Read the model definition and answer for the solid it produces. Units are mm, in the model's axes. A direction names the side the tool comes from. Give positions to 0.01 mm unless a question says otherwise; leave off trailing zeros. Order: outer loops, then holes, each group sorted by start corner. A loop starts at its lowest first (then second) coordinate and runs counter-clockwise, first axis right, second up. Notation, with made-up numbers: (9.25, 60) -> (34.25, 60) arc R11 cw to (34.25, 64) -> close; hole circle Ø6 at (86.25, 68.5). An arc over 180 degrees is marked (long way). Use one line per item in the form item = value.
```python
from build123d import *

# Parameters (mm, degrees)
SKETCH_1_R                   = 2.6
SM_BASE_FLANGE_1_DEPTH       = 1.2
SM_EDGE_FLANGE_2_DEPTH       = 160
SM_START                     = 1.2
SM_EDGE_FLANGE_2_PROFILE_R   = 5
SM_EDGE_FLANGE_2_PROFILE_R_2 = 2.6
SM_EDGE_FLANGE_2_FLAT_DEPTH  = 1.2


# Sheet-metal steps are written as plain solids
with BuildPart() as part:
    # Sketch 1 → 基体-法兰1 (new body)
    with BuildSketch(Plane.XY):
        with BuildLine():
            Line((-8, 80), (9, 80))
            Line((9, 80), (9, -80))
            Line((9, -80), (-8, -80))
            ThreePointArc((-8, -80), (-9.414213562, -79.414213562), (-10, -78))
            Line((-10, -78), (-10, 78))
            ThreePointArc((-10, 78), (-9.414213562, 79.414213562), (-8, 80))
        make_face()
        with Locations((0, 70)):
            Circle(SKETCH_1_R, mode=Mode.SUBTRACT)
        with Locations((0, -70)):
            Circle(SKETCH_1_R, mode=Mode.SUBTRACT)
    extrude(amount=-SM_BASE_FLANGE_1_DEPTH)

    # 边线-法兰2 bend section (across the edge) → 边线-法兰2 (add)
    with BuildSketch(Plane(origin=(10, -80, 0), x_dir=(-1, 0, 0), z_dir=(0, 1, 0))):
        with BuildLine():
            Line((-1.2, 1), (0, 1))
            ThreePointArc((0, 1), (0.292893219, 0.292893219), (1, 0))
            Line((1, 0), (1, -1.2))
            ThreePointArc((1, -1.2), (-0.555634919, -0.555634919), (-1.2, 1))
        make_face()
    extrude(amount=SM_EDGE_FLANGE_2_DEPTH)

    # 边线-法兰2 profile (on flange) → 边线-法兰2 flat (add)
    with BuildSketch(Plane.YZ.offset(10).offset(SM_START)):
        with BuildLine():
            Line((-80, 15), (-80, 1))
            Line((-80, 1), (80, 1))
            Line((80, 1), (80, 15))
            ThreePointArc((80, 15), (78.535533906, 18.535533906), (75, 20))
            Line((75, 20), (-75, 20))
            ThreePointArc((-75, 20), (-78.535533906, 18.535533906), (-80, 15))
        make_face()
        with Locations((-70, 10)):
            Circle(SM_EDGE_FLANGE_2_PROFILE_R, mode=Mode.SUBTRACT)
        with Locations((0, 10)):
            Circle(SM_EDGE_FLANGE_2_PROFILE_R_2, mode=Mode.SUBTRACT)
        with Locations((70, 10)):
            Circle(SM_EDGE_FLANGE_2_PROFILE_R, mode=Mode.SUBTRACT)
    extrude(amount=-SM_EDGE_FLANGE_2_FLAT_DEPTH)


solid = part.part
```
Item 1: The part is cut by section D-D on x = -0.75. Give the vertices of the cut face in (y, z).
Checks:
outline = (-80, -1.2) -> (-72.49, -1.2) -> (-72.49, 0) -> (-80, 0) -> close; (-67.51, -1.2) -> (67.51, -1.2) -> (67.51, 0) -> (-67.51, 0) -> close; (72.49, -1.2) -> (80, -1.2) -> (80, 0) -> (72.49, 0) -> close
Item 2: Given pin 1 Ø6 at (x, y) = (1.5, -8.5) entering from +Z; pin 2 Ø4 at (x, z) = (6.5, 15.5) entering from +Y; pin 3 Ø12 at (y, z) = (18.5, 11) entering from -X, each flat-ended and moving along its own axis, determine where each tip first touches the part or whether it passes through.
Checks:
pin_1 = 0
pin_2 = through
pin_3 = 10
Item 3: The part is cut by section A-A on y = -70. Give the vertices of the cut face in (x, z), and give its area (3 significant figures).
Checks:
outline = (-10, -1.2) -> (-2.6, -1.2) -> (-2.6, 0) -> (-10, 0) -> close; (2.6, -1.2) -> (9, -1.2) arc R2.2 ccw to (11.2, 1) -> (11.2, 5) -> (10, 5) -> (10, 1) arc R1 cw to (9, 0) -> (2.6, 0) -> close; (10, 15) -> (11.2, 15) -> (11.2, 20) -> (10, 20) -> close
area = 30.4 mm²
Item 4: Which of the six approach directions +Z, -Z, +X, -X, +Y, -Y give full straight-line access (tool end or side, diameter ignored) to faces 1 (the flat face through (11.2, -1, 13)), 2 (the flat face through (0, 1, 0))?
Checks:
face_1 = +Z, -Z, +X, +Y, -Y
face_2 = +Z, -X, +Y, -Y
Item 5: Determine the mould class of faces 3 (the cylindrical face through (11, 79, 18)), 4 (the cylindrical face through (-0.338, 72.578, -0.592)), 5 (the flat face through (5.9, -80, -0.3)), 6 (the flat face through (10, -1, 13)) for opening direction Y: +Y half, -Y half, draft (parallel to the pull), parting line (faces both ways), or undercut.
Checks:
face_3 = +Y half
face_4 = undercut
face_5 = -Y half
face_6 = draft
Item 6: Straight lines are drawn through the part: L1, parallel to Y at x = 0, z = -0.75; L2, parallel to X at y = -31, z = 1.25; L3, parallel to Z at x = -5, y = -15. For each, find the intervals that lie inside material, in ascending order. Write a range as from..to.
Checks:
L1 = -80..-72.6, -67.4..67.4, 72.6..80
L2 = 10..11.2
L3 = -1.2..0
Item 7: The part is cut by section C-C on y = 0. Give the vertices of the cut face in (x, z), and give its area (3 significant figures).
Checks:
outline = (-10, -1.2) -> (9, -1.2) arc R2.2 ccw to (11.2, 1) -> (11.2, 7.4) -> (10, 7.4) -> (10, 1) arc R1 cw to (9, 0) -> (-10, 0) -> close; (10, 12.6) -> (11.2, 12.6) -> (11.2, 20) -> (10, 20) -> close
area = 42.4 mm²
Item 8: The part is cut by section B-B on z = 10. Give the vertices of the cut face in (x, y).
Checks:
outline = (10, -80) -> (11.2, -80) -> (11.2, -75) -> (10, -75) -> close; (10, -65) -> (11.2, -65) -> (11.2, -2.6) -> (10, -2.6) -> close; (10, 2.6) -> (11.2, 2.6) -> (11.2, 65) -> (10, 65) -> close; (10, 75) -> (11.2, 75) -> (11.2, 80) -> (10, 80) -> close
